CAD build for the part. Positions are in the model's coordinates, mm. A direction names the side the tool comes from. Coordinates: 2 decimals unless noted, no trailing zeros. Loops run counter-clockwise (first coordinate to the right, second up) from the corner with the lowest first, then second, coordinate; pieces in that order, holes last. Notation, with made-up numbers: (78.25, -34.5) -> (128.25, -34.5) arc R27 cw to (128.25, -14.5) -> close; hole circle Ø11 at (-29, 1.5). An arc over 180 degrees is marked (long way). Answer as CSV lines item,"result". Start each with the question number.
from build123d import *

# Parameters (mm, degrees)
SKETCH_1_R      = 12.5
EXTRUDE_1_DEPTH = 50


with BuildPart() as part:
    # Эскиз1 → Бобышка-Вытянуть1 (new body)
    with BuildSketch(Plane.XY):
        with BuildLine():
            Line((-3.5, 18.206279241), (-3.5, 20.706279241))
            ThreePointArc((-3.5, 20.706279241), (-18.186533479, 10.5), (-19.68216384, -7.322050707))
            Line((-19.68216384, -7.322050707), (-17.517100331, -6.072050707))
            Line((-17.517100331, -6.072050707), (-14.017100331, -12.134228534))
            Line((-14.017100331, -12.134228534), (-16.18216384, -13.384228534))
            ThreePointArc((-16.18216384, -13.384228534), (0, -21), (16.18216384, -13.384228534))
            Line((16.18216384, -13.384228534), (14.017100331, -12.134228534))
            Line((14.017100331, -12.134228534), (17.517100331, -6.072050707))
            Line((17.517100331, -6.072050707), (19.68216384, -7.322050707))
            ThreePointArc((19.68216384, -7.322050707), (20.667915239, -3.719849416), (21, 0))
            ThreePointArc((21, 0), (16.039014932, 13.555441712), (3.5, 20.706279241))
            Line((3.5, 20.706279241), (3.5, 18.206279241))
            Line((3.5, 18.206279241), (-3.5, 18.206279241))
        make_face()
        Circle(SKETCH_1_R, mode=Mode.SUBTRACT)
    extrude(amount=EXTRUDE_1_DEPTH)


solid = part.part
Item 1: Saw through at C-C (z = 42). Write the cut outline in (x, y), plus the area to 3 significant figures.
Item 2: Saw through at A-A (x = 0). Write the cut outline in (y, z), plus the area to 3 significant figures.
Item 3: Two-plate mould, pull along X, no slides. Class faces 5 (the face through (11.923, 3.755, 24.65)), 6 (the face through (-18.06, 10.72, 24.65)), 7 (the face through (9, -9, 0)): pulls with the +X half, pulls with the -X half, needs draft (parallel to the pull), parting line crosses it, or undercut.
Item 4: Which spindle directions (+Z, -Z, +X, -X, +Y, -Y) get a long thin tool onto all of the face, cutting with end or side? Do faces 1 (the face through (-18.615, -6.706, 24.65)), 2 (the face through (15.74, -9.15, 24.65)), 3 (the face through (0, 18.206, 25)), 4 (the face through (15.115, -12.768, 24.65)). Say none if no direction does.
Item 5: Saw through at B-B (y = 1). Write the cut outline in (x, z).
Item 6: Saw through at D-D (y = 14). Write the cut outline in (x, z), plus the area to 3 significant figures.
Item 7: Flat gauge pins, fed straight in: pin 1 Ø10 at (x, z) = (-3, 17) entering from +Y; pin 2 Ø2 at (x, z) = (-1.5, 20) entering from +Y; pin 3 Ø1 at (y, z) = (-9, 14.5) entering from +X. Where does each tip first touch, or does it go through?
Item 8: Wall check: probe 1 along Y at (x, z) = (0, 30); probe 2 along X at (y, z) = (6.5, 35); probe 3 along X at (y, z) = (9, 46). Give the ranges that are in metal, low to high.
Geometry check:
1,outline,"(-19.68, -7.32) -> (-17.52, -6.07) -> (-14.02, -12.13) -> (-16.18, -13.38) arc R21 ccw to (16.18, -13.38) -> (14.02, -12.13) -> (17.52, -6.07) -> (19.68, -7.32) arc R21 ccw to (3.5, 20.71) -> (3.5, 18.21) -> (-3.5, 18.21) -> (-3.5, 20.71) arc R21 ccw to start; hole circle Ø25 at (0, 0)"
1,area,"838 mm2"
2,outline,"(-21, 0) -> (-12.5, 0) -> (-12.5, 50) -> (-21, 50) -> close; (12.5, 0) -> (18.21, 0) -> (18.21, 50) -> (12.5, 50) -> close"
2,area,"710 mm2"
3,face 5,"undercut"
3,face 6,"pulls with the -X half"
3,face 7,"needs draft"
4,face 1,"+Z, -Z, -Y"
4,face 2,"+Z, -Z"
4,face 3,"+Z, -Z, +Y"
4,face 4,"+Z, -Z, +X"
5,outline,"(-20.98, 0) -> (-12.46, 0) -> (-12.46, 50) -> (-20.98, 50) -> close; (12.46, 0) -> (20.98, 0) -> (20.98, 50) -> (12.46, 50) -> close"
6,outline,"(-15.65, 0) -> (15.65, 0) -> (15.65, 50) -> (-15.65, 50) -> close"
6,area,"1,570 mm2"
7,pin 1,"y = 20.71"
7,pin 2,"y = 18.21"
7,pin 3,"x = 16.12"
8,probe 1,"-21 to -12.5, 12.5 to 18.21"
8,probe 2,"-19.97 to -10.68, 10.68 to 19.97"
8,probe 3,"-18.97 to -8.67, 8.67 to 18.97"
